Here's how the part is built. I have some questions about the finished solid (model axes, mm). Face numbers are marked on the shaded views. A direction names the side the tool comes from. Round coordinates to 2 decimals unless told otherwise and drop trailing zeros. Loops run counter-clockwise (first coordinate to the right, second up) from the corner with the lowest first, then second, coordinate; pieces in that order, holes last. Notation, with made-up numbers: (88, 27) -> (120, 27) arc R20 cw to (120, 38) -> close; hole circle Ø9 at (54, -8.75). An arc over 180 degrees is marked (long way). Use one line per item in the form item = value. Start each with the question number.
Item 1: I'm going to push flat-ended pins straight in: pin 1 Ø1 at (y, z) = (15.5, -40.5) entering from -X; pin 2 Ø10.5 at (x, y) = (-16.5, -10.5) entering from -Z; pin 3 Ø8 at (x, z) = (9.5, 24.5) entering from -Y; pin 4 Ø8.5 at (x, z) = (-39.37, 0) entering from -Y. Where does each tip first touch, or does it pass through?
Item 2: For the marked faces 4, 5, 6 and 7, which set-ups out of +Z, -Z, +X, -X, +Y, -Y let a thin tool reach every point of the face, with its end or its side?
Item 3: If we section it at C-C (x = 5.5): Write out the boundary of the cut face in (y, z) (3 decimals), then the cut area to 3 significant figures.
Item 4: If we section it at A-A (z = 0): State how many separate pieces and enclosed holes the cut face has, then the cut area to 3 significant figures.
Item 5: If I drill on L1, parallel to Z at x = -16, y = -21; L2, parallel to X at y = -18.25, z = 0 (3 decimals); L3, parallel to Z at x = -1, y = 8 (3 decimals), over which ranges is the centre line in solid material (lowest first)? Write a range as [from, to].
Item 6: Thinking about a two-plate mould opening in Z: for the marked faces 1, 2 and 3, which applies, released by +Z, released by -Z, zero draft, split by the parting line, or undercut?
Item 7: If we section it at B-B (y = -7.5): Write out the boundary of the cut face in (x, z) (1 decimal), then the cut area to 3 significant figures.
```python
from build123d import *

# Parameters (mm, degrees)
BOSS_EXTRUDE1_DEPTH   = 23.495
FILLET1_R             = 25.4
SHELL1_T              = -4.445
NUB_DEPTH             = 23.368
FILLET2_R             = 12.7
FILLET3_R             = 6.858
CUT_EXTRUDE1_DEPTH    = 21.463
CHAMFER1_SIZE         = 1.016
BOSS_EXTRUDE2_DEPTH   = 23.495
F_8_CLEARANCE_HOLE1_D = 4.4958
CHAMFER2_SIZE         = 1.016
SKETCH14_R            = 3.675
CUT_EXTRUDE2_DEPTH    = 122.72544216


with BuildPart() as part:
    # Sketch1 → Boss-Extrude1 (new body)
    with BuildSketch(Plane(origin=(0, 0, 0), x_dir=(1, 0, 0), z_dir=(0, 1, 0))):
        with BuildLine():
            Line((-25.4, -76.2), (69.85, -76.2))
            Line((69.85, -76.2), (69.85, 76.2))
            Line((69.85, 76.2), (-25.4, 76.2))
            Line((-25.4, 76.2), (-49.305882353, 31.376470588))
            ThreePointArc((-49.305882353, 31.376470588), (-57.15, 0), (-49.305882353, -31.376470588))
            Line((-49.305882353, -31.376470588), (-25.4, -76.2))
        make_face()
    extrude(amount=BOSS_EXTRUDE1_DEPTH)

    # Fillet1
    fillet1_edges = [part.edges().sort_by_distance(p)[0] for p in [
        (69.85, 11.7475, 76.2),
        (-25.4, 11.7475, 76.2),
        (-25.4, 11.7475, -76.2),
        (69.85, 11.7475, -76.2),
    ]]
    fillet(fillet1_edges, radius=FILLET1_R)

    # Shell1
    shell1_openings = [part.faces().sort_by_distance(p)[0] for p in [
        (11.569703313, 23.495, 0),
    ]]
    offset(amount=SHELL1_T, openings=shell1_openings, kind=Kind.INTERSECTION)

    # Sketch13 → nub (add)
    with BuildSketch(Plane.XZ):
        with BuildLine():
            Line((-2.54, 38.1), (-2.54, -38.1))
            Line((-2.54, -38.1), (-40.216666667, -38.1))
            Line((-40.216666667, -38.1), (-44.599411765, -29.882352941))
            ThreePointArc((-44.599411765, -29.882352941), (-52.07, 0), (-44.599411765, 29.882352941))
            Line((-44.599411765, 29.882352941), (-40.216666667, 38.1))
            Line((-40.216666667, 38.1), (-2.54, 38.1))
        make_face()
    extrude(amount=NUB_DEPTH)

    # Fillet2
    fillet2_edges = [part.edges().sort_by_distance(p)[0] for p in [
        (-40.216666667, -11.684, 38.1),
        (-40.216666667, -11.684, -38.1),
    ]]
    fillet(fillet2_edges, radius=FILLET2_R)

    # Fillet3
    fillet3_edges = [part.edges().sort_by_distance(p)[0] for p in [
        (-2.54, -11.684, 38.1),
        (-2.54, -11.684, -38.1),
    ]]
    fillet(fillet3_edges, radius=FILLET3_R)

    # Sketch8 → Cut-Extrude1 (cut)
    with BuildSketch(Plane(origin=(0, 4.445, 0), x_dir=(1, 0, 0), z_dir=(0, 1, 0))):
        with BuildLine():
            Line((-32.596666667, -33.655), (-9.398, -33.655))
            ThreePointArc((-9.398, -33.655), (-7.691751337, -32.948248663), (-6.985, -31.242))
            Line((-6.985, -31.242), (-6.985, 31.242))
            ThreePointArc((-6.985, 31.242), (-7.691751337, 32.948248663), (-9.398, 33.655))
            Line((-9.398, 33.655), (-32.596666667, 33.655))
            ThreePointArc((-32.596666667, 33.655), (-36.843829128, 32.478604102), (-39.880490196, 29.284705882))
            Line((-39.880490196, 29.284705882), (-40.677352941, 27.790588235))
            ThreePointArc((-40.677352941, 27.790588235), (-47.625, 0), (-40.677352941, -27.790588235))
            Line((-40.677352941, -27.790588235), (-39.880490196, -29.284705882))
            ThreePointArc((-39.880490196, -29.284705882), (-36.843829128, -32.478604102), (-32.596666667, -33.655))
        make_face()
    extrude(amount=-CUT_EXTRUDE1_DEPTH, mode=Mode.SUBTRACT)

    # Chamfer1
    chamfer1_edges = [part.edges().sort_by_distance(p)[0] for p in [
        (-37.016764706, 23.495, 44.972941176),
        (-20.941258555, 23.495, 68.768764258),
        (17.145, 23.495, 71.755),
        (59.2674226, 23.495, 65.6174226),
        (65.405, 23.495, 0),
        (59.2674226, 23.495, -65.6174226),
        (17.145, 23.495, -71.755),
        (-20.941258555, 23.495, -68.768764258),
        (-37.016764706, 23.495, -44.972941176),
        (-52.705, 23.495, 0),
    ]]
    chamfer(chamfer1_edges, length=CHAMFER1_SIZE)

    # Sketch10 → Boss-Extrude2 (add)
    with BuildSketch(Plane(origin=(0, 23.495, 0), x_dir=(1, 0, 0), z_dir=(0, 1, 0))):
        with BuildLine():
            Line((69.85, 47.625), (69.85, 15.875))
            ThreePointArc((69.85, 15.875), (72.024192281, 22.073146175), (77.593902439, 25.554878049))
            ThreePointArc((77.593902439, 25.554878049), (82.55, 31.75), (77.593902439, 37.945121951))
            ThreePointArc((77.593902439, 37.945121951), (72.024192281, 41.426853825), (69.85, 47.625))
        make_face()
        with BuildLine():
            Line((69.85, -47.625), (69.85, -15.875))
            ThreePointArc((69.85, -15.875), (72.024192281, -22.073146175), (77.593902439, -25.554878049))
            ThreePointArc((77.593902439, -25.554878049), (82.55, -31.75), (77.593902439, -37.945121951))
            ThreePointArc((77.593902439, -37.945121951), (72.024192281, -41.426853825), (69.85, -47.625))
        make_face()
        with BuildLine():
            Line((-33.069803922, 61.819117647), (-48.010980392, 33.804411765))
            ThreePointArc((-48.010980392, 33.804411765), (-47.012610676, 40.296513581), (-50.288598757, 45.989670014))
            ThreePointArc((-50.288598757, 45.989670014), (-51.74627451, 53.788235294), (-44.457895744, 56.922238164))
            ThreePointArc((-44.457895744, 56.922238164), (-37.904983546, 57.373314449), (-33.069803922, 61.819117647))
        make_face()
        with BuildLine():
            Line((-33.069803922, -61.819117647), (-48.010980392, -33.804411765))
            ThreePointArc((-48.010980392, -33.804411765), (-47.012610676, -40.296513581), (-50.288598757, -45.989670014))
            ThreePointArc((-50.288598757, -45.989670014), (-51.74627451, -53.788235294), (-44.457895744, -56.922238164))
            ThreePointArc((-44.457895744, -56.922238164), (-37.904983546, -57.373314449), (-33.069803922, -61.819117647))
        make_face()
    extrude(amount=-BOSS_EXTRUDE2_DEPTH)

    # #8 Clearance Hole1 (through all)
    with Locations(Plane(origin=(0, 23.495, 0), x_dir=(-1, 0, 0), z_dir=(0, 1, 0))):
        with Locations((46.143333333, -50.8), (46.143333333, 50.8), (-76.2, 31.75), (-76.2, -31.75)):
            Hole(F_8_CLEARANCE_HOLE1_D / 2)

    # Chamfer2
    chamfer2_edges = [part.edges().sort_by_distance(p)[0] for p in [
        (-20.997333333, -23.368, 38.1),
        (-4.548661695, -23.368, 36.091338305),
        (-4.548661695, -23.368, -36.091338305),
        (69.85, 0, -49.2125),
        (72.024192281, 0, -22.073146175),
        (82.55, 0, -31.75),
        (72.024192281, 0, -41.426853825),
        (69.85, 0, 0),
        (72.024192281, 0, 22.073146175),
        (72.024192281, 0, 41.426853825),
        (82.55, 0, 31.75),
        (17.145, 0, 76.2),
        (-48.658431373, 0, -32.590441176),
        (-51.74627451, 0, -53.788235294),
        (-47.012610676, 0, -40.296513581),
        (-37.904983546, 0, -57.373314449),
        (-32.820784314, 0, 62.286029412),
        (-47.012610676, 0, 40.296513581),
        (-51.74627451, 0, 53.788235294),
        (-37.904983546, 0, 57.373314449),
        (69.85, 0, 49.2125),
        (-32.820784314, 0, -62.286029412),
        (17.145, 0, -76.2),
        (-23.228192188, 0, -72.580320313),
        (62.410512242, 0, -68.760512242),
        (62.410512242, 0, 68.760512242),
        (-23.228192188, 0, 72.580320313),
        (-48.658431373, 0, 32.590441176),
        (-57.15, 0, 0),
        (-52.07, -23.368, 0),
        (-44.200980392, -23.368, -30.629411765),
        (-20.997333333, -23.368, -38.1),
        (-44.200980392, -23.368, 30.629411765),
        (-39.130762761, -23.368, 36.290160157),
        (-39.130762761, -23.368, -36.290160157),
        (-2.54, -23.368, 0),
    ]]
    chamfer(chamfer2_edges, length=CHAMFER2_SIZE)

    # Sketch14 → Cut-Extrude2 (cut, through all)
    with BuildSketch(Plane.XZ.offset(23.368)):
        with Locations(Location((-16.51, 22.86, 0), (0, 0, 270))):
            Circle(SKETCH14_R)
        with Locations(Location((-16.51, 0, 0), (0, 0, 270))):
            Circle(SKETCH14_R)
        with Locations(Location((-16.51, -22.86, 0), (0, 0, 270))):
            Circle(SKETCH14_R)
        with Locations(Location((-39.37, 0, 0), (0, 0, 270))):
            Circle(SKETCH14_R)
    extrude(amount=-CUT_EXTRUDE2_DEPTH, mode=Mode.SUBTRACT)


solid = part.part
```
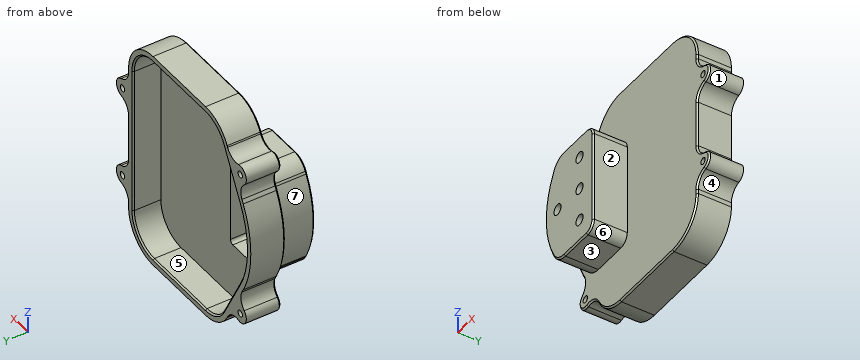
Values found:
q1.pin_1 = -47.17
q1.pin_2 = -38.1
q1.pin_3 = 0
q1.pin_4 = -23.37
q2.face_4 = -Z, +X, +Y, -Y
q2.face_5 = +Y
q2.face_6 = -Z, +X, -Y
q2.face_7 = -X, -Y
q3.outline = (0, -75.184) -> (1.016, -76.2) -> (23.495, -76.2) -> (23.495, -72.771) -> (22.479, -71.755) -> (4.445, -71.755) -> (4.445, 71.755) -> (22.479, 71.755) -> (23.495, 72.771) -> (23.495, 76.2) -> (1.016, 76.2) -> (0, 75.184) -> close
q3.area = 845 mm2
q4.separate_pieces = 3
q4.enclosed_holes = 0
q4.area = 923 mm2
q5.L1 = [-38.1, -26.5], [-19.22, -3.64], [3.64, 19.22], [26.5, 38.1]
q5.L2 = [-52.07, -43.045], [-35.695, -20.185], [-12.835, -2.54]
q5.L3 = [-76.2, -71.755], [71.755, 76.2]
q6.face_1 = undercut
q6.face_2 = zero draft
q6.face_3 = released by -Z
q7.outline = (-44.6, -29.9) -> (-43.8, -31.4) arc R12.7 ccw to (-32.6, -38.1) -> (-9.4, -38.1) arc R6.9 ccw to (-2.5, -31.2) -> (-2.5, 31.2) arc R6.9 ccw to (-9.4, 38.1) -> (-32.6, 38.1) arc R12.7 ccw to (-43.8, 31.4) -> (-44.6, 29.9) arc R63.5 ccw to start; hole (-40.7, -27.8) -> (-39.9, -29.3) arc R8.3 ccw to (-32.6, -33.7) -> (-9.4, -33.7) arc R2.4 ccw to (-7, -31.2) -> (-7, 31.2) arc R2.4 ccw to (-9.4, 33.7) -> (-32.6, 33.7) arc R8.3 ccw to (-39.9, 29.3) -> (-40.7, 27.8) arc R59.1 ccw to start
q7.area = 931 mm2
